```python
from build123d import *

# Parameters (mm, degrees)
SKETCH2_W                         = 28
SKETCH2_H                         = 60
BOSS_EXTRUDE1_DEPTH               = 290
SKETCH3_W                         = 8
SKETCH3_H                         = 16
CUT_EXTRUDE1_DEPTH                = 581.944059269
CHAMFER1_SIZE                     = 10
FILLET1_R                         = 5
M10X1_25_TAPPED_HOLE1_D           = 8.8
M10X1_25_TAPPED_HOLE1_CSINK_D     = 10.05
M10X1_25_TAPPED_HOLE1_CSINK_ANGLE = 90
LPATTERN1_COUNT                   = 5
LPATTERN1_PITCH                   = 132.5


with BuildPart() as part:
    # Sketch2 → Boss-Extrude1 (new, symmetric)
    with BuildSketch(Plane(origin=(0, 0, 0), x_dir=(-1, 0, 0), z_dir=(0, 1, 0))):
        Rectangle(SKETCH2_W, SKETCH2_H)
    extrude(amount=BOSS_EXTRUDE1_DEPTH, both=True)

    # Sketch3 → Cut-Extrude1 (cut, through all)
    with BuildSketch(Plane(origin=(0, 290, 0), x_dir=(-1, 0, 0), z_dir=(0, 1, 0))):
        with Locations((-10, 7)):
            Rectangle(SKETCH3_W, SKETCH3_H)
    extrude(amount=-CUT_EXTRUDE1_DEPTH, mode=Mode.SUBTRACT)

    # Chamfer1
    chamfer1_edges = [part.edges().sort_by_distance(p)[0] for p in [
        (14, 0, -30),
    ]]
    chamfer(chamfer1_edges, length=CHAMFER1_SIZE)

    # Fillet1
    fillet1_edges = [part.edges().sort_by_distance(p)[0] for p in [
        (-14, 0, -30),
    ]]
    fillet(fillet1_edges, radius=FILLET1_R)

    # M10x1.25 Tapped Hole1 (through all)
    with Locations(Plane.YZ.offset(6)):
        with Locations((-265, 7)):
            m10x1_25_tapped_hole1 = CounterSinkHole(M10X1_25_TAPPED_HOLE1_D / 2, M10X1_25_TAPPED_HOLE1_CSINK_D / 2, counter_sink_angle=M10X1_25_TAPPED_HOLE1_CSINK_ANGLE)

    # LPattern1: M10x1.25 Tapped Hole1 ×5
    with Locations(*[(0, i * LPATTERN1_PITCH, 0) for i in range(1, LPATTERN1_COUNT)]):
        add(m10x1_25_tapped_hole1, mode=Mode.SUBTRACT)


solid = part.part
```
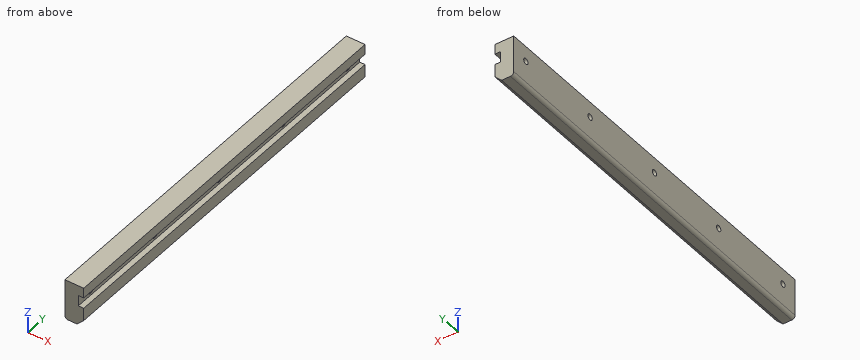
Can you work these out from the model? Positions are in its coordinate system, mm. Give positions to 0.01 mm unless a question says otherwise; leave off trailing zeros. Order: outer loops, then holes, each group sorted by start corner. A loop starts at its lowest first (then second) coordinate and runs counter-clockwise, first axis right, second up. Notation, with made-up numbers: (-34, -12.75) - (-25, -12.75) arc R20 cw to (-25, 12.25) - close; hole circle Ø9 at (7.25, 77.5). An arc over 180 degrees is marked (long way). Use a Markdown table: item, result. Add a question column.
Q1. I'm going to push flat-ended pins straight in: pin 1 (7 mm diameter, centred on y = 0, z = 7, fed in from -X); pin 2 (8 mm diameter, centred on y = -58.5, z = 8.5, fed in from +X); pin 3 (9 mm diameter, centred on x = 10, y = 84, fed in from -Z). Where does each tip first touch, or does it pass through?
Q2. If we section it at A-A on y = -89.5: Write out the boundary of the cut face in (x, z).
Q3. Please list where these lines run through material, in increasing order: line 1 along Y through (x, z) = (-7, 7); line 2 along Y through (x, z) = (5.5, 6.5); line 3 along Z through (x, y) = (-6.25, 132.5).
Answers follow:
| question | item | result |
|---|---|---|
| 1 | pin 1 | passes through |
| 1 | pin 2 | stops at x = 6 |
| 1 | pin 3 | stops at z = -28.5 |
| 2 | outline | (-14, -25) arc R5 ccw to (-9, -30) - (4, -30) - (14, -20) - (14, -1) - (6, -1) - (6, 15) - (14, 15) - (14, 30) - (-14, 30) - close |
| 3 | line 1 | y = -290 to -269.4, -260.6 to -136.9, -128.1 to -4.4, 4.4 to 128.1, 136.9 to 260.6, 269.4 to 290 |
| 3 | line 2 | y = -290 to -269.5, -260.5 to -137, -128 to -4.5, 4.5 to 128, 137 to 260.5, 269.5 to 290 |
| 3 | line 3 | z = -30 to 2.6, 11.4 to 30 |
